from build123d import *

# Parameters (mm, degrees)
F1_DEPTH = 5
F2_R     = 1.45235
F3_DEPTH = 26
F5_R     = 1.8
F6_DEPTH = 25


with BuildPart() as f1:
    # F0 (on Front) → F1 (new body, symmetric)
    with BuildSketch(Plane.XZ):
        Polygon((53.554079, -3.796815), (-20.445921, -3.796815), (-26.445921, -3.796815), (-26.445921, -21.796815), (-20.445921, -21.796815), (53.554079, -21.796815), align=None)
        with BuildLine():
            Line((97.775743, 19.536518), (53.554079, -3.796815))
            Line((53.554079, -3.796815), (53.554079, -21.796815))
            ThreePointArc((53.554079, -21.796815), (58.625986, -21.023499), (63.236974, -18.773824))
            Line((63.236974, -18.773824), (106.620076, 6.203185))
            Line((106.620076, 6.203185), (97.775743, 19.536518))
        make_face()
        with BuildLine():
            ThreePointArc((101.961013, 24.4677), (100.137325, 21.773844), (97.775743, 19.536518))
            Line((97.775743, 19.536518), (106.620076, 6.203185))
            ThreePointArc((106.620076, 6.203185), (113.834838, 12.659729), (117.171564, 21.748515))
            Line((117.171564, 21.748515), (115.640686, 41.689839))
            Line((115.640686, 41.689839), (100.812855, 39.423693))
            Line((100.812855, 39.423693), (101.961013, 24.4677))
        make_face()
        Polygon((93.643953, 46.395555), (100.812855, 39.423693), (115.640686, 41.689839), (101.302883, 55.633563), (99.707273, 53.708978), (98.743672, 52.546706), (97.148061, 50.622121), (95.239564, 48.32014), align=None)
        Polygon((89.794783, 49.586776), (93.643953, 46.395555), (95.239564, 48.32014), (91.390394, 51.511361), align=None)
        Polygon((99.707273, 53.708978), (101.302883, 55.633563), (97.453713, 58.824784), (95.858103, 56.900199), align=None)
        Polygon((93.298891, 53.813342), (97.148061, 50.622121), (98.743672, 52.546706), (94.894502, 55.737927), align=None)
    extrude(amount=F1_DEPTH, both=True)

    # F2 (on face) → F3 (cut)
    with BuildSketch(Plane.XZ.offset(5)):
        with Locations((30.503755, -13.683314)):
            Circle(F2_R)
    extrude(amount=-F3_DEPTH, mode=Mode.SUBTRACT)

    # F5 (on face) → F6 (cut)
    with BuildSketch(Plane.XZ.offset(5)):
        with Locations((-22.781451, -12.652125)):
            Circle(F5_R)
    extrude(amount=-F6_DEPTH, mode=Mode.SUBTRACT)


solid = f1.part
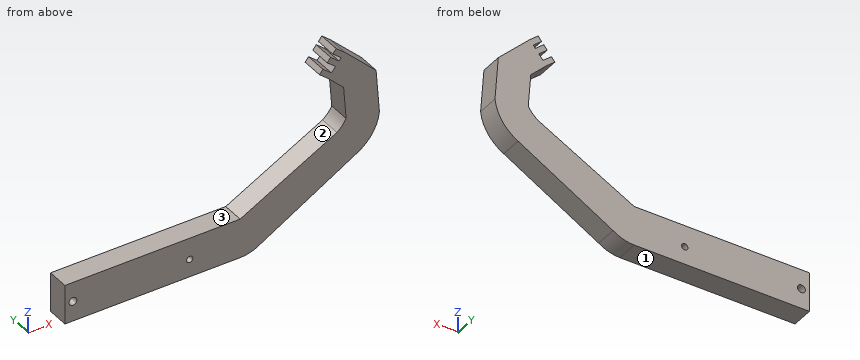
Can you work these out from the model? Positions are in its coordinate system, mm. Face numbers are marked on the shaded views. A direction names the side the tool comes from. Round coordinates to 2 decimals unless told otherwise and drop trailing zeros. Loops run counter-clockwise (first coordinate to the right, second up) from the corner with the lowest first, then second, coordinate; pieces in that order, holes last. Notation, with made-up numbers: (23.25, -23.75) - (27.25, -23.75) arc R30 ccw to (27.25, 0.25) - close; hole circle Ø3 at (37, 66.25). An arc over 180 degrees is marked (long way). Answer in a Markdown table with one row per item. Add a question column.
Q1. I want a section at B-B on x = -15. List the corners of the cut face in (y, z) for me.
Q2. I want a section at A-A on y = 2.5. List the corners of the cut face in (x, z) for me.
Q3. I want a section at C-C on z = 35.5. List the corners of the cut face in (x, y) for me, and give its area (3 significant figures).
Q4. Which directions (+Z, -Z, +X, -X, +Y, -Y) give clear straight access to the entire face, cutting with the end or side of a thin tool? Please do the marked faces 1, 2 and 3.
Q5. I need wall thicknesses on L1, parallel to Z at x = -19, y = 3; L2, parallel to X at y = 0, z = 50; L3, parallel to X at y = -4, z = 51. Which ranges of each line are inside material? Lowest first, please.
Q6. For pin 1 Ø1 at (x, y) = (50, -1.5) entering from +Z; pin 2 Ø1.5 at (x, y) = (56.5, 4) entering from -Z; pin 3 Ø2 at (y, z) = (0, 45.5) entering from -X; pin 4 Ø2.5 at (x, z) = (30.5, -13.68) entering from +Y, each with a flat end and sliding along its axis, tell me the tip position at first contact or that it passes through.
A:
| question | item | result |
|---|---|---|
| 1 | outline | (-5, -21.8) - (5, -21.8) - (5, -3.8) - (-5, -3.8) - close |
| 2 | outline | (-26.45, -21.8) - (53.55, -21.8) arc R17.02 ccw to (63.24, -18.77) - (106.62, 6.2) arc R20 ccw to (117.17, 21.75) - (115.64, 41.69) - (101.3, 55.63) - (97.45, 58.82) - (95.86, 56.9) - (99.71, 53.71) - (98.74, 52.55) - (94.89, 55.74) - (93.3, 53.81) - (97.15, 50.62) - (95.24, 48.32) - (91.39, 51.51) - (89.79, 49.59) - (93.64, 46.4) - (100.81, 39.42) - (101.96, 24.47) arc R15 cw to (97.78, 19.54) - (53.55, -3.8) - (-26.45, -3.8) - close; hole circle Ø3.6 at (-22.78, -12.65); hole circle Ø2.9 at (30.5, -13.68) |
| 3 | outline | (101.11, -5) - (116.12, -5) - (116.12, 5) - (101.11, 5) - close |
| 3 | area | 150 mm^2 |
| 4 | face 1 | -Z, +X, -X, +Y, -Y |
| 4 | face 2 | -X, +Y, -Y |
| 4 | face 3 | +Z, -X, +Y, -Y |
| 5 | L1 | -21.8 to -3.8 |
| 5 | L2 | 90.14 to 93.21, 96.63 to 107.1 |
| 5 | L3 | 90.97 to 92.01, 96.69 to 106.07 |
| 6 | pin 1 | z = -3.8 |
| 6 | pin 2 | z = -21.65 |
| 6 | pin 3 | x = 93.52 |
| 6 | pin 4 | through |
